from build123d import *

# Parameters (mm, degrees)
SKETCH1_W                 = 50
SKETCH1_H                 = 40
BOSS_EXTRUDE1_DEPTH       = 100
SKETCH2_W                 = 30
SKETCH2_H                 = 30
CUT_EXTRUDE1_DEPTH        = 100
SKETCH3_R                 = 3.5
CUT_EXTRUDE2_DEPTH        = 10
M5X0_8_TAPPED_HOLE1_D     = 4.2
M5X0_8_TAPPED_HOLE1_DEPTH = 14
M5X0_8_TAPPED_HOLE1_TIP   = 1.2618073
M5X0_8_TAPPED_HOLE2_D     = 4.2
M5X0_8_TAPPED_HOLE2_DEPTH = 14
M5X0_8_TAPPED_HOLE2_TIP   = 1.2618073
M5X0_8_TAPPED_HOLE3_D     = 4.2
M5X0_8_TAPPED_HOLE3_DEPTH = 14
M5X0_8_TAPPED_HOLE3_TIP   = 1.2618073
M5X0_8_TAPPED_HOLE4_D     = 4.2
M5X0_8_TAPPED_HOLE4_DEPTH = 14
M5X0_8_TAPPED_HOLE4_TIP   = 1.2618073


with BuildPart() as part:
    # Sketch1 → Boss-Extrude1 (new body)
    with BuildSketch(Plane(origin=(0, 0, 0), x_dir=(1, 0, 0), z_dir=(0, 1, 0))):
        Rectangle(SKETCH1_W, SKETCH1_H)
    extrude(amount=BOSS_EXTRUDE1_DEPTH)

    # Sketch2 → Cut-Extrude1 (cut)
    with BuildSketch(Plane(origin=(0, 100, 0), x_dir=(1, 0, 0), z_dir=(0, 1, 0))):
        with Locations((0, -5)):
            Rectangle(SKETCH2_W, SKETCH2_H)
    extrude(amount=-CUT_EXTRUDE1_DEPTH, mode=Mode.SUBTRACT)

    # Sketch3 → Cut-Extrude2 (cut)
    with BuildSketch(Plane(origin=(0, 0, -20), x_dir=(-1, 0, 0), z_dir=(0, 0, -1))):
        with Locations((0, 25)):
            Circle(SKETCH3_R)
        with Locations((0, 75)):
            Circle(SKETCH3_R)
    extrude(amount=-CUT_EXTRUDE2_DEPTH, mode=Mode.SUBTRACT)

    # M5x0.8 Tapped Hole1
    with Locations(Plane.XZ):
        with Locations((0, -15), (-20, 5), (20, 5)):
            Hole(M5X0_8_TAPPED_HOLE1_D / 2, depth=M5X0_8_TAPPED_HOLE1_DEPTH)
            with Locations((0, 0, -(M5X0_8_TAPPED_HOLE1_DEPTH + M5X0_8_TAPPED_HOLE1_TIP / 2))):  # 118° drill point
                Cone(0, M5X0_8_TAPPED_HOLE1_D / 2, M5X0_8_TAPPED_HOLE1_TIP, mode=Mode.SUBTRACT)

    # M5x0.8 Tapped Hole2
    with Locations(Plane(origin=(0, 100, 0), x_dir=(-1, 0, 0), z_dir=(0, 1, 0))):
        with Locations((20, 5), (-20, 5), (0, -15)):
            Hole(M5X0_8_TAPPED_HOLE2_D / 2, depth=M5X0_8_TAPPED_HOLE2_DEPTH)
            with Locations((0, 0, -(M5X0_8_TAPPED_HOLE2_DEPTH + M5X0_8_TAPPED_HOLE2_TIP / 2))):  # 118° drill point
                Cone(0, M5X0_8_TAPPED_HOLE2_D / 2, M5X0_8_TAPPED_HOLE2_TIP, mode=Mode.SUBTRACT)

    # M5x0.8 Tapped Hole3
    with Locations(Plane(origin=(25, 0, 0), x_dir=(0, 0, -1), z_dir=(1, 0, 0))):
        with Locations((15, 75), (15, 25)):
            Hole(M5X0_8_TAPPED_HOLE3_D / 2, depth=M5X0_8_TAPPED_HOLE3_DEPTH)
            with Locations((0, 0, -(M5X0_8_TAPPED_HOLE3_DEPTH + M5X0_8_TAPPED_HOLE3_TIP / 2))):  # 118° drill point
                Cone(0, M5X0_8_TAPPED_HOLE3_D / 2, M5X0_8_TAPPED_HOLE3_TIP, mode=Mode.SUBTRACT)

    # M5x0.8 Tapped Hole4
    with Locations(Plane.ZY.offset(25)):
        with Locations((-15, 75), (-15, 25)):
            Hole(M5X0_8_TAPPED_HOLE4_D / 2, depth=M5X0_8_TAPPED_HOLE4_DEPTH)
            with Locations((0, 0, -(M5X0_8_TAPPED_HOLE4_DEPTH + M5X0_8_TAPPED_HOLE4_TIP / 2))):  # 118° drill point
                Cone(0, M5X0_8_TAPPED_HOLE4_D / 2, M5X0_8_TAPPED_HOLE4_TIP, mode=Mode.SUBTRACT)


solid = part.part
Verification items for the finished model (mm, model axes). A direction names the side the tool comes from. Coordinates: 2 decimals unless noted, no trailing zeros. Write each loop counter-clockwise with the first axis right and the second up, starting at its lowest first coordinate (ties: lowest second). Pieces come first, ordered by that corner, then holes. Notation, with made-up numbers: M -37,-19 L -11,-19 A31 cw -11,20 Z; hole C 18.5,12.25 d5. An arc over 180 degrees is marked long. Use CSV: the item, a comma, the result in double quotes.
Q1. Mould release check, pull along X, two halves, no side actions. Record for faces 1 (the conical face through (-0.047, 15.043, -14.638)), 2 (the conical face through (9.96, 24.64, -14.92)), 3 (the cylindrical face through (-17.9, 26.77, -16.13)): pulls with the +X half, pulls with the -X half, needs draft (parallel to the pull), parting line crosses it, or undercut.
Computed values:
face 1,"undercut"
face 2,"pulls with the +X half"
face 3,"needs draft"
Q2. Section check B-B, the plane y = 11.5. Enter the section's corners in (x, z), and give its area (3 significant figures).
Computed values:
outline,"M -25,-20 L 25,-20 L 25,20 L 15,20 L 15,-10 L -15,-10 L -15,20 L -25,20 Z; hole C -20,5 d4.2; hole C 0,-15 d4.2; hole C 20,5 d4.2"
area,"1,060 mm²"
Q3. Section check A-A, the plane z = -7. Enter the section's corners in (x, y).
Computed values:
outline,"M -25,0 L -15,0 L -15,100 L -25,100 Z; M 15,0 L 25,0 L 25,100 L 15,100 Z"
Q4. Thickness scan on line 1 along Y through (x, z) = (-15.75, -15); line 2 along X through (y, z) = (3, 5); line 3 along X through (y, z) = (86, -8). Record the ranges inside material, lowest first. Write a range as [from, to].
Computed values:
line 1,"[0, 22.9], [27.1, 72.9], [77.1, 100]"
line 2,"[-25, -22.1], [-17.9, -15], [15, 17.9], [22.1, 25]"
line 3,"[-25, -15], [15, 25]"
Q5. Section check C-C, the plane y = 46. Enter the section's corners in (x, z), and give its area (3 significant figures).
Computed values:
outline,"M -25,-20 L 25,-20 L 25,20 L 15,20 L 15,-10 L -15,-10 L -15,20 L -25,20 Z"
area,"1,100 mm²"
Q6. Section check D-D, the plane x = -8.5. Enter the section's corners in (y, z).
Computed values:
outline,"M 0,-20 L 100,-20 L 100,-10 L 0,-10 Z"
Q7. Set-up check for faces 4 (the cylindrical face through (-17.902, 76.419, -13.452)), 5 (the cylindrical face through (22.003, 92.902, 5.631)), 6 (the cylindrical face through (17.997, 7.098, 5.631)), 7 (the flat face through (0, 51, -10)): record each of +Z, -Z, +X, -X, +Y, -Y from which the full face is reachable in a straight line by a thin tool's end or side.
Computed values:
face 4,"-X"
face 5,"+Y"
face 6,"-Y"
face 7,"+Z, +Y, -Y"
Q8. Go/stop test with flat-tipped pins: P1, Ø6.5, axis at y = 75, z = -15, coming from the +X side; P2, Ø2.5, axis at x = 20, z = 5, coming from the -Y side; P3, Ø9, axis at x = 7, y = 56, coming from the +Z side; P4, Ø3.5, axis at y = 25, z = -15, coming from the +X side. Record where each tip stops, or that it passes through.
Computed values:
P1,"x = 25"
P2,"y = 14.51"
P3,"z = -10"
P4,"x = 10.79"
